Source: CAD feature listing. Evaluate the final solid. Frame: model axes, mm. A direction names the side the tool comes from. Coordinates: 2 decimals unless noted, no trailing zeros. Order: outer loops, then holes, each group sorted by start corner. A loop starts at its lowest first (then second) coordinate and runs counter-clockwise, first axis right, second up.
Autodesk Inventor part; units mm, degrees
ref_plane "XZ Plane" through (0, 0, 0) normal (0, 1, 0) x (-1, 0, 0)
ref_plane "XY Plane" through (0, 0, 0) normal (0, 0, 1) x (1, 0, 0)
sketch "Boceto1" plane through (0, 0, 0) normal (0, 0, 1) x (1, 0, 0)
  line L0 (0, 0) -> (39, 0) construction
  line L1 (39, 0) -> (39, 35)
  line L2 (39, 35) -> (43, 35)
  line L3 (43, 35) -> (43, 42)
  arc A0 (48, 47) -> (43, 42) centre (48, 42) ccw
  line L4 (48, 47) -> (48, 229)
  line L5 (0, 0) -> (0, 229) construction
  line L6 (48, 229) -> (44, 229)
  line L7 (0, 112) -> (48, 112) construction
  line L8 (48, 112) -> (48, 77) construction
  line L9 (48, 77) -> (48, 56) construction
  line L10 (44, 229) -> (44, 56)
  line L11 (44, 56) -> (40, 56)
  line L12 (40, 56) -> (40, 65)
  line L13 (40, 65) -> (35, 60)
  line L14 (39, 0) -> (35, 0)
  line L15 (35, 0) -> (35, 60)
  dimension "d0" = 39
  dimension "d1" = 35
  dimension "d2" = 4
  dimension "d7" = 5
  dimension "d9" = 229
  dimension "d10" = 12
  dimension "d11" = 5
  dimension "d12" = 182
  dimension "d13" = 4
  dimension "d14" = 117
  dimension "d15" = 35
  dimension "d16" = 21
  dimension "d17" = 4
  dimension "d18" = 9
  dimension "d19" = 45
  dimension "d20" = 4
  dimension "d21" = 173
revolve "Revolución1" add sketch "Boceto1" angle 360 about axis through (0, 0, 0) along (0, 1, 0)
sketch "Boceto2" plane through (0, 0, 0) normal (0, 0, 1) x (1, 0, 0)
  line L0 (48, 229) -> (-48, 229)
  line L1 (48, 47) -> (-48, 47)
  line L2 (39, 35) -> (-39, 35)
  line L3 (39, 0) -> (-39, 0)
  line L4 (0, 0) -> (0, 112) construction
  line L5 (0, 112) -> (101, 112) construction
  dimension "d23" = 112
  dimension "d24" = 101
ref_plane "Plano de trabajo1" through (101, 112, 0) normal (1, 0, 0) x (0, 1, 0)
sketch "Boceto3" plane through (101, 112, 0) normal (1, 0, 0) x (0, 1, 0)
  circle A0 centre (0, 0) radius 39
  point P0 (-112, 0)
  dimension "d25" = 78
  dimension "d26" = 112
extrude "Extrusión1" add sketch "Boceto3" against normal up to surface
sketch "Boceto4" plane through (101, 112, 0) normal (1, 0, 0) x (0, 0, -1)
  circle A0 centre (0, 0) radius 35
  circle A1 centre (0, 0) radius 39
  point P0 (0, -112)
  dimension "d29" = 70
  dimension "d30" = 4
extrude "Extrusión2" cut sketch "Boceto4" against normal up to surface contours A0
properties part number "7_Cuerpo"
Q1. Set-up query: faces 4 (the flat face through (10, 56, 39)), 5 (the cylindrical face through (73.114, 83.255, 26.358)), 6 (the cylindrical face through (-5.598, 38.549, -42.634)), 7 (the flat face through (21, 229, 39)). Return all of +Z, -Z, +X, -X, +Y, -Y with unobstructed straight access to the full face (end or side cutting, diameter ignored); none if empty.
Solutions:
face 4: +Y
face 5: +X
face 6: -Y
face 7: +Z, -Z, +X, -X, +Y
Q2. Pull-direction query (Y, two-part tool) for faces 1 (the flat face through (9.35, 35, 38.02)), 2 (the cylindrical face through (72.61, 122.513, -33.384)), 3 (the conical face through (33.68, 60.31, -10.61)); classes: pulls with the +Y half, pulls with the -Y half, needs draft (parallel to the pull), parting line crosses it, or undercut.
Solutions:
face 1: pulls with the -Y half
face 2: undercut
face 3: pulls with the +Y half
Q3. Material intervals for line 1 along Z through (x, y) = (45, 112); line 2 along Z through (x, y) = (0, 136), sorted ascending.
Solutions:
line 1: z = -39 to -35, 35 to 39
line 2: z = -48 to -44, 44 to 48
Q4. Section query B-B on x = 0. Output: boundary loops of the cut face in (y, z), plus the area to 3 significant figures.
Solutions:
outline: (0, -39) - (35, -39) - (35, -43) - (42, -43) arc R5 cw to (47, -48) - (229, -48) - (229, -44) - (56, -44) - (56, -40) - (65, -40) - (60, -35) - (0, -35) - close; (0, 35) - (60, 35) - (65, 40) - (56, 40) - (56, 44) - (229, 44) - (229, 48) - (47, 48) arc R5 cw to (42, 43) - (35, 43) - (35, 39) - (0, 39) - close
area: 2,170 mm2
Q5. Section query C-C on y = 112. Output: boundary loops of the cut face in (x, z).
Solutions:
outline: (26.66, -35) arc R44 cw (long way) to (26.66, 35) - (101, 35) - (101, 39) - (27.98, 39) arc R48 ccw (long way) to (27.98, -39) - (101, -39) - (101, -35) - close
Q6. Section query D-D on y = 180. Output: boundary loops of the cut face in (x, z), plus the area to 3 significant figures.
Solutions:
outline: circle Ø96 at (0, 0); hole circle Ø88 at (0, 0)
area: 1,160 mm2
Q7. Pin query (flat end, axial travel): P1, Ø8, axis at y = 189.5, z = -31, coming from the -X side; P2, Ø3, axis at x = -18.5, y = 129.5, coming from the -Z side; P3, Ø1.5, axis at x = 35, z = -7.5, coming from the +Y side. Return the tip coordinate at first contact, or that it passes through.
Solutions:
P1: stops at x = -39.69
P2: stops at z = -44.89
P3: stops at y = 61.54
Q8. Section query A-A on z = 0. Give the number of separate pieces and of enclosed holes in the cut face, plus the area to 3 significant figures.
Solutions:
separate pieces: 3
enclosed holes: 0
area: 2,310 mm2
